from build123d import *

# Parameters (mm, degrees)
F1_DEPTH = 9
F2_R     = 6.5
F3_DEPTH = 5
F5_DEPTH = 5
F6_R     = 2
F8_DEPTH = 5


with BuildPart() as f1:
    # F0 (on Right) → F1 (new body)
    with BuildSketch(Plane.YZ):
        with BuildLine():
            Line((0, -207.12592), (0, 0))
            Line((0, 0), (-80, 29.117619))
            Line((-80, 29.117619), (-80, -150))
            ThreePointArc((-80, -150), (-72.766082, -172.943057), (-53.680806, -187.587705))
            Line((-53.680806, -187.587705), (0, -207.12592))
        make_face()
    extrude(amount=F1_DEPTH)

    # F2 (on face) → F3 (cut)
    with BuildSketch(Plane(origin=(0, 0, 0), x_dir=(0, -1, 0), z_dir=(-1, 0, 0))):
        with Locations((40, -150)):
            Circle(F2_R)
    extrude(amount=-F3_DEPTH, mode=Mode.SUBTRACT)

    # F4 (on face) → F5 (cut)
    with BuildSketch(Plane(origin=(0, 0, 0), x_dir=(0, -1, 0), z_dir=(-1, 0, 0))):
        Polygon((75, -57.836454), (5, -83.314371), (5, -88.635259), (75, -63.157343), align=None)
    extrude(amount=-F5_DEPTH, mode=Mode.SUBTRACT)

    # F6
    f6_edges = [f1.edges().sort_by_distance(p)[0] for p in [
        (4.5, 0, -207.12592),
        (4.5, -80, 29.117619),
    ]]
    fillet(f6_edges, radius=F6_R)

    # F7 (on face) → F8 (cut)
    with BuildSketch(Plane(origin=(0, 0, 0), x_dir=(0, -1, 0), z_dir=(-1, 0, 0))):
        Polygon((3.5, -80), (3.5, 1.273896), (0, 0), (0, -80), align=None)
    extrude(amount=-F8_DEPTH, mode=Mode.SUBTRACT)


solid = f1.part
Design review of the part built by this model. Coordinates are the model's own, in mm. A direction names the side the tool comes from. Coordinates: 2 decimals unless noted, no trailing zeros. Write each loop counter-clockwise with the first axis right and the second up, starting at its lowest first coordinate (ties: lowest second). Pieces come first, ordered by that corner, then holes. Notation, with made-up numbers: (38, 67) - (94, 67) arc R18 ccw to (94, 86) - close; hole circle Ø2 at (56, 57). An arc over 180 degrees is marked (long way). One line per item, written item: value.
1) Insertion check: pin 1 (1 mm diameter, centred on x = 4, y = -23.5, fed in from -Z); pin 2 (2.5 mm diameter, centred on x = 2, z = -39, fed in from +Y); pin 3 (1 mm diameter, centred on x = 2, y = -2, fed in from +Z). Each pin has a flat end and moves straight along its axis. Give the tip position at first contact, or say it passes through.
Answer sheet:
pin 1: stops at z = -198.75
pin 2: stops at y = -3.5
pin 3: stops at z = -80
2) For faces 4 (the face through (4, 0, -126)), 5 (the face through (2, -3.5, -40)), 6 (the face through (2.465, -39.51, -76.075)), list the 3-axis set-ups (+Z, -Z, +X, -X, +Y, -Y) from which the entire face can be reached by the end or side of a thin tool; tool diameter is ignored.
Answer sheet:
face 4: +Z, -Z, +X, -X, +Y
face 5: +Z, -X, +Y
face 6: -X
3) Add section B-B (y = -14). State the section outline as (x, z) points.
Answer sheet:
outline: (0, -202.03) - (9, -202.03) - (9, 5.1) - (0, 5.1) - (0, -80.04) - (5, -80.04) - (5, -85.36) - (0, -85.36) - close
4) Mouldability with a two-part tool opening along Z and no side actions: class faces 1 (the face through (5, -40, -73)), 2 (the face through (9, -41, -87)), 3 (the face through (4.437, -38.117, 13.873)) as +Z half, -Z half, draft (parallel to the pull), parting line (faces both ways), or undercut.
Answer sheet:
face 1: undercut
face 2: draft
face 3: +Z half
5) Add section A-A (x = 7.25). State the section outline as (y, z) points, plus the area to 3 significant figures.
Answer sheet:
outline: (-80, -150) arc R40 ccw to (-53.68, -187.59) - (-2.68, -206.15) arc R2 ccw to (0, -204.27) - (0, 0) - (-77.32, 28.14) arc R2 ccw to (-80, 26.26) - close
area: 16,400 mm2
6) Add section C-C (z = 9). State the section outline as (x, y) points, plus the area to 3 significant figures.
Answer sheet:
outline: (0, -80) - (9, -80) - (9, -24.73) - (0, -24.73) - close
area: 497 mm2
7) Add section D-D (y = -38.5). State the section outline as (x, z) points.
Answer sheet:
outline: (0, -193.11) - (9, -193.11) - (9, 14.01) - (0, 14.01) - (0, -71.12) - (5, -71.12) - (5, -76.44) - (0, -76.44) - (0, -143.68) - (5, -143.68) - (5, -156.32) - (0, -156.32) - close
8) To check wall thickness, follow probe 1 along Z at (x, y) = (3.95, -40); probe 2 along Y at (x, z) = (0.75, -12); probe 3 along Z at (x, y) = (3, -17.5). State the ranges of each line that lie inside material, in increasing order.
Answer sheet:
probe 1: z = -192.57 to -156.5, -143.5 to -75.9, -70.58 to 14.56
probe 2: y = -80 to -3.5
probe 3: z = -200.76 to -84.09, -78.76 to 6.37
